from build123d import *

# Parameters (mm, degrees)
SALIENTE_EXTRUIR2_DEPTH = 19
CROQUIS3_R              = 2.5
SALIENTE_EXTRUIR3_DEPTH = 1.5
CROQUIS4_R              = 2
CORTAR_EXTRUIR1_DEPTH   = 0.5
CROQUIS5_R              = 1
SALIENTE_EXTRUIR4_DEPTH = 8.5
SALIENTE_EXTRUIR5_START = 5
SALIENTE_EXTRUIR5_DEPTH = 5
SALIENTE_EXTRUIR6_DEPTH = 2
CORTAR_EXTRUIR2_START   = -0.01
CROQUIS8_R              = 2
CORTAR_EXTRUIR2_DEPTH   = 0.01
SALIENTE_EXTRUIR7_START = 0.9
CROQUIS9_R              = 1
SALIENTE_EXTRUIR7_DEPTH = 0.9
CROQUIS10_W             = 7
CROQUIS10_H             = 1.5
SALIENTE_EXTRUIR8_DEPTH = 5


with BuildPart() as part:
    # Croquis2 → Saliente-Extruir2 (new body)
    with BuildSketch(Plane.XY):
        with BuildLine():
            Line((-7, 7.5), (7, 7.5))
            ThreePointArc((7, 7.5), (10.259142264, 0), (7, -7.5))
            Line((7, -7.5), (-7, -7.5))
            ThreePointArc((-7, -7.5), (-10.259142264, 0), (-7, 7.5))
        make_face()
    extrude(amount=SALIENTE_EXTRUIR2_DEPTH)

    # Croquis3 → Saliente-Extruir3 (add)
    with BuildSketch(Plane.XY.offset(19)):
        Circle(CROQUIS3_R)
    extrude(amount=SALIENTE_EXTRUIR3_DEPTH)

    # Croquis4 → Cortar-Extruir1 (cut)
    with BuildSketch(Plane.XY.offset(20.5)):
        Circle(CROQUIS4_R)
    extrude(amount=-CORTAR_EXTRUIR1_DEPTH, mode=Mode.SUBTRACT)

    # Croquis5 → Saliente-Extruir4 (add)
    with BuildSketch(Plane.XY.offset(20)):
        Circle(CROQUIS5_R)
    extrude(amount=SALIENTE_EXTRUIR4_DEPTH)

    # Croquis6 → Saliente-Extruir5 (add)
    with BuildSketch(Plane(origin=(0, 0, 0), x_dir=(-1, 0, 0), z_dir=(0, 0, -1)).offset(SALIENTE_EXTRUIR5_START)):
        with BuildLine():
            Line((-7, 7.5), (7, 7.5))
            ThreePointArc((7, 7.5), (9.332754717, 4.260245227), (10.252272727, 0.375371717))
            ThreePointArc((10.252272727, 0.375371717), (7.3, 0), (10.252272727, -0.375371717))
            ThreePointArc((10.252272727, -0.375371717), (9.332754717, -4.260245227), (7, -7.5))
            Line((7, -7.5), (-7, -7.5))
            ThreePointArc((-7, -7.5), (-9.332754717, -4.260245227), (-10.252272727, -0.375371717))
            ThreePointArc((-10.252272727, -0.375371717), (-7.3, 0), (-10.252272727, 0.375371717))
            ThreePointArc((-10.252272727, 0.375371717), (-9.332754717, 4.260245227), (-7, 7.5))
        make_face()
    extrude(amount=-SALIENTE_EXTRUIR5_DEPTH)

    # Croquis7 → Saliente-Extruir6 (add)
    with BuildSketch(Plane(origin=(0, 0, -5), x_dir=(-1, 0, 0), z_dir=(0, 0, -1))):
        with BuildLine():
            Line((-3, -3.354101966), (3, -3.354101966))
            ThreePointArc((3, -3.354101966), (0, 4.5), (-3, -3.354101966))
        make_face()
    extrude(amount=SALIENTE_EXTRUIR6_DEPTH)

    # Croquis8 → Cortar-Extruir2 (cut)
    with BuildSketch(Plane(origin=(0, 0, -7), x_dir=(-1, 0, 0), z_dir=(0, 0, -1)).offset(CORTAR_EXTRUIR2_START)):
        with Locations(Location((0, 0, 0), (0, 0, 180))):
            Circle(CROQUIS8_R)
    extrude(amount=CORTAR_EXTRUIR2_DEPTH, mode=Mode.SUBTRACT)

    # Croquis9 → Saliente-Extruir7 (add)
    with BuildSketch(Plane(origin=(0, 0, -6.99), x_dir=(-1, 0, 0), z_dir=(0, 0, -1)).offset(SALIENTE_EXTRUIR7_START)):
        with Locations(Location((0, 0, 0), (0, 0, 180))):
            Circle(CROQUIS9_R)
    extrude(amount=-SALIENTE_EXTRUIR7_DEPTH)

    # Croquis10 → Saliente-Extruir8 (add)
    with BuildSketch(Plane(origin=(0, 0, -5), x_dir=(-1, 0, 0), z_dir=(0, 0, -1))):
        with Locations((0, 8.25)):
            Rectangle(CROQUIS10_W, CROQUIS10_H)
    extrude(amount=-SALIENTE_EXTRUIR8_DEPTH)


solid = part.part
Here's how the part is built. I have some questions about the finished solid (model axes, mm). A direction names the side the tool comes from. Round coordinates to 2 decimals unless told otherwise and drop trailing zeros. Write each loop counter-clockwise with the first axis right and the second up, starting at its lowest first coordinate (ties: lowest second). Pieces come first, ordered by that corner, then holes.
1. If we mould it in two halves opening along Y, with no side actions, what happens to faces 1 (the flat face through (-9, 0, 0)), 2 (the flat face through (-3.5, 8, -3)), 3 (the flat face through (0, 9, -3))? For each: released by +Y, released by -Y, zero draft, split by the parting line, or undercut.
2. Suppose I cut it at B-B (z = -4). List the corners of the cut face in (x, y) for me, and give its area (3 significant figures).
3. For faces 4 (the flat face through (0, -3.354, -6)), 5 (the cylindrical face through (7.3, -0.06, -2.54)), 6 (the flat face through (-2, -2, 19)), which set-ups out of +Z, -Z, +X, -X, +Y, -Y let a thin tool reach every point of the face, with its end or its side?
4. I need wall thicknesses on L1, parallel to Y at x = 0, z = 20.1; L2, parallel to Z at x = -7.25, y = -2; L3, parallel to X at y = 0, z = -1.7. Which ranges of each line are inside material? Lowest first, please.
5. Suppose I cut it at D-D (x = -8.8). List the corners of the cut face in (y, z) for me, and give its area (3 significant figures).
6. Will these pins go through, and if not, where does the flat tip stop? pin 1 Ø3 at (y, z) = (-2, 18) entering from -X; pin 2 Ø3.5 at (x, y) = (8.5, 0.5) entering from -Z; pin 3 Ø4 at (x, z) = (1.5, 12) entering from +Y.
Answer sheet:
1. face 1: undercut
1. face 2: zero draft
1. face 3: released by +Y
2. outline: (-10.25, -0.38) arc R10.26 ccw to (-7, -7.5) - (7, -7.5) arc R10.26 ccw to (10.25, -0.38) arc R1.5 cw (long way) to (10.25, 0.38) arc R10.26 ccw to (7, 7.5) - (3.5, 7.5) - (3.5, 9) - (-3.5, 9) - (-3.5, 7.5) - (-7, 7.5) arc R10.26 ccw to (-10.25, 0.38) arc R1.5 cw (long way) to start
2. area: 274 mm2
3. face 4: -Z, +X, -X, -Y
3. face 5: -Z
3. face 6: +Z
4. L1: y = -2.5 to -2, -1 to 1, 2 to 2.5
4. L2: z = -5 to 19
4. L3: x = -7.3 to 7.3
5. outline: (-5.27, -5) - (-1.5, -5) - (-1.5, 0) - (1.5, 0) - (1.5, -5) - (5.27, -5) - (5.27, 19) - (-5.27, 19) - close
5. area: 238 mm2
6. pin 1: stops at x = -10.25
6. pin 2: stops at z = -5
6. pin 3: stops at y = 7.5
